The model under review builds one solid part; all positions refer to its coordinate system, in mm. A direction names the side the tool comes from. Round coordinates to 2 decimals unless told otherwise and drop trailing zeros. Write each loop counter-clockwise with the first axis right and the second up, starting at its lowest first coordinate (ties: lowest second). Pieces come first, ordered by that corner, then holes.
Item 1: Add section A-A (z = 20.75). Give the boundary of the cut face in (x, y), plus the area to 3 significant figures.
Item 2: Add section C-C (y = 2.5). Give the boundary of the cut face in (x, z), plus the area to 3 significant figures.
Item 3: Add section D-D (x = -53). Give the boundary of the cut face in (y, z).
Item 4: To check wall thickness, follow L1, parallel to Y at x = -59.75, z = 10.5; L2, parallel to Z at x = -66, y = 1.75; L3, parallel to X at y = -2, z = 17.5. State the ranges of each line that lie inside material, in increasing order.
Item 5: Add section B-B (x = -70.5). Give the boundary of the cut face in (y, z), plus the area to 3 significant figures.
Item 6: Machinability: for faces 1 (the face through (-51.17, 5, 18)), 2 (the face through (-76.04, 4.93, 18.13)), 3 (the face through (-54, 5, 19.214)), 4 (the face through (-54, 5, 16.214)), 5 (the face through (-60.7, 0, 17.6)), which of the approach directions +Z, -Z, +X, -X, +Y, -Y give a long, thin tool a straight path to every point of the face, cutting with its end or side? Answer none if there is none.
Item 7: Clearance check with flat-ended pins moving along their axes: pin 1 Ø4 at (x, y) = (-63, 6) entering from +Z; pin 2 Ø5 at (y, z) = (-6, 22) entering from +X; pin 3 Ø3 at (y, z) = (5.5, 14) entering from +X. State where each tip first meets the part, or that it passes through.
```python
from build123d import *

# Parameters (mm, degrees)
SKETCH1_R           = 5
BOSS_EXTRUDE1_DEPTH = 10
SKETCH1_3_R         = 5
BOSS_EXTRUDE2_DEPTH = 10


with BuildPart() as part:
    # Sketch1 → Boss-Extrude1 (new body)
    with BuildSketch(Plane(origin=(0, 0, 0), x_dir=(1, 0, 0), z_dir=(0, 1, 0))):
        with BuildLine():
            Line((-56.169981336, -16.214278262), (-51.169981336, -16.214278262))
            Line((-51.169981336, -16.214278262), (-51.169981336, -19.214278262))
            Line((-51.169981336, -19.214278262), (-56.169981336, -19.214278262))
            ThreePointArc((-56.169981336, -19.214278262), (-76.049815498, -17.714278262), (-56.169981336, -16.214278262))
        make_face()
        with Locations((-66.053308407, -17.714278262)):
            Circle(SKETCH1_R, mode=Mode.SUBTRACT)
        with Locations((-66.053308407, -17.714278262)):
            Circle(SKETCH1_R)
    extrude(amount=BOSS_EXTRUDE1_DEPTH)

    # Sketch1_3 → Boss-Extrude2 (add)
    with BuildSketch(Plane(origin=(0, 0, 0), x_dir=(1, 0, 0), z_dir=(0, 1, 0))):
        with Locations((-66.053308407, -17.714278262)):
            Circle(SKETCH1_3_R)
    extrude(amount=-BOSS_EXTRUDE2_DEPTH)


solid = part.part
```
Numbers:
1. outline: (-75.58, 0) - (-70.03, 0) - (-70.03, -10) - (-62.08, -10) - (-62.08, 0) - (-56.53, 0) - (-56.53, 10) - (-75.58, 10) - close
1. area: 270 mm2
2. outline: (-56.17, 16.21) - (-51.17, 16.21) - (-51.17, 19.21) - (-56.17, 19.21) arc R10 ccw (long way) to start
2. area: 329 mm2
3. outline: (0, 16.21) - (10, 16.21) - (10, 19.21) - (0, 19.21) - close
4. L1: y = 0 to 10
4. L2: z = 7.72 to 27.71
4. L3: x = -71.05 to -61.06
5. outline: (-10, 15.43) - (0, 15.43) - (0, 8.76) - (10, 8.76) - (10, 26.67) - (0, 26.67) - (0, 20) - (-10, 20) - close
5. area: 225 mm2
6. face 1: +Z, -Z, +X, +Y, -Y
6. face 2: +Y, -Y
6. face 3: +Z, +X, +Y, -Y
6. face 4: -Z, +X, +Y, -Y
6. face 5: -Y
7. pin 1: stops at z = 27.66
7. pin 2: stops at x = -61.38
7. pin 3: stops at x = -56.31
